from build123d import *

# Parameters (mm, degrees)
CROQUIS1_W              = 70
CROQUIS1_H              = 90
SALIENTE_EXTRUIR1_DEPTH = 3
CROQUIS2_R              = 1
CORTAR_EXTRUIR1_DEPTH   = 3
CHAFL_N1_START          = 47.29332687
CHAFL_N1_OUTLINE_W      = 17
CHAFL_N1_OUTLINE_H      = 5
CHAFL_N1_DEPTH          = 7.70667313
CHAFL_N2_START          = -48
CHAFL_N2_OUTLINE_W      = 17
CHAFL_N2_OUTLINE_H      = 5
CHAFL_N2_DEPTH          = 7.713379536
CROQUIS4_W              = 66.199172227
CROQUIS4_H              = 50.611167931
SALIENTE_EXTRUIR2_DEPTH = 3
CROQUIS5_R              = 0.75
CORTAR_EXTRUIR2_DEPTH   = 67.497809415


with BuildPart() as part:
    # Croquis1 → Saliente-Extruir1 (new body)
    with BuildSketch(Plane.XY):
        with Locations((4.954489614, -8.071625344)):
            Rectangle(CROQUIS1_W, CROQUIS1_H)
    extrude(amount=SALIENTE_EXTRUIR1_DEPTH)

    # Croquis2 → Cortar-Extruir1 (cut)
    with BuildSketch(Plane(origin=(0, 0, 0), x_dir=(-1, 0, 0), z_dir=(0, 0, -1))):
        with Locations((-34.954489614, -49.571625344)):
            Circle(CROQUIS2_R)
        with Locations((25.045510386, -49.571625344)):
            Circle(CROQUIS2_R)
        with Locations((-34.954489614, -6.571625344)):
            Circle(CROQUIS2_R)
        with Locations((25.045510386, -6.571625344)):
            Circle(CROQUIS2_R)
    extrude(amount=-CORTAR_EXTRUIR1_DEPTH, mode=Mode.SUBTRACT)

    # Chafl_n1: read off the stored shape, not the designer's step
    # Chafl_n1 outline → Chafl_n1 (cut)
    with BuildSketch(Plane(origin=(0, 0, 0), x_dir=(0.707106781186548, -0.707106781186547, 0), z_dir=(0.707106781186547, 0.707106781186548, 0)).offset(CHAFL_N1_START)):
        with Locations((2.5, -1.5)):
            Rectangle(CHAFL_N1_OUTLINE_W, CHAFL_N1_OUTLINE_H)
    extrude(amount=CHAFL_N1_DEPTH, mode=Mode.SUBTRACT)

    # Chafl_n2: read off the stored shape, not the designer's step
    # Chafl_n2 outline → Chafl_n2 (cut)
    with BuildSketch(Plane(origin=(0, 0, 0), x_dir=(0.7071067811865474, 0.7071067811865477, 0), z_dir=(0.7071067811865476, -0.7071067811865476, 0)).offset(CHAFL_N2_START)):
        with Locations((4.5, 1.5)):
            Rectangle(CHAFL_N2_OUTLINE_W, CHAFL_N2_OUTLINE_H)
    extrude(amount=CHAFL_N2_DEPTH, mode=Mode.SUBTRACT)

    # Croquis4 → Saliente-Extruir2 (add)
    with BuildSketch(Plane.XY.offset(3)):
        with Locations((4.57620863, -27.766041379)):
            Rectangle(CROQUIS4_W, CROQUIS4_H)
    extrude(amount=-SALIENTE_EXTRUIR2_DEPTH)

    # Croquis5 → Cortar-Extruir2 (cut, through all)
    with BuildSketch(Plane.XY.offset(3)):
        with Locations((-10.045510386, 1.928374656)):
            Circle(CROQUIS5_R)
        with Locations((19.954489614, 1.928374656)):
            Circle(CROQUIS5_R)
        with Locations((-10.045510386, -49.071625344)):
            Circle(CROQUIS5_R)
        with Locations((19.954489614, -49.071625344)):
            Circle(CROQUIS5_R)
    extrude(amount=-CORTAR_EXTRUIR2_DEPTH, mode=Mode.SUBTRACT)


solid = part.part
Read the model definition and answer for the solid it produces. Units are mm, in the model's axes. Coordinates: 2 decimals unless noted, no trailing zeros. Write each loop counter-clockwise with the first axis right and the second up, starting at its lowest first coordinate (ties: lowest second). Pieces come first, ordered by that corner, then holes. Notation, with made-up numbers: (88, -36) - (117, -36) arc R14 cw to (117, -17) - close; hole circle Ø9 at (19.5, -37). An arc over 180 degrees is marked (long way). One line per question, with ' | ' between items.
Q1. Find section B-B, the plane y = 30.5. Write down the section's boundary in (x, z).
Result set:
outline: (-26.47, 0) - (36.38, 0) - (36.38, 3) - (-26.47, 3) - close
Q2. Find section A-A, the plane z = 2.3. Write down the section's boundary in (x, y), plus the area to 3 significant figures.
Result set:
outline: (-30.05, -53.07) - (39.95, -53.07) - (39.95, 26.93) - (29.95, 36.93) - (-20.05, 36.93) - (-30.05, 26.93) - close; hole circle Ø1.5 at (-10.05, -49.07); hole circle Ø1.5 at (-10.05, 1.93); hole circle Ø1.5 at (19.95, -49.07); hole circle Ø1.5 at (19.95, 1.93) | area: 6,190 mm^2
Q3. Consider L1, parallel to Y at x = 37.5, z = 0.8; L2, parallel to Y at x = 30, z = 1.65. Determine where each line is inside the solid, lowest interval first. Write a range as [from, to].
Result set:
L1: [-53.07, 29.38] | L2: [-53.07, 36.88]
Q4. This flat-tipped pin is pushed along its axis until it touches: P1, Ø0.9, axis at x = -10.05, y = -49.07, coming from the +Z side. Where does it stop, or does it pass through?
Result set:
P1: through
